The model under review builds one solid part; all positions refer to its coordinate system, in mm. A direction names the side the tool comes from. Give positions to 0.01 mm unless a question says otherwise; leave off trailing zeros. Write each loop counter-clockwise with the first axis right and the second up, starting at its lowest first coordinate (ties: lowest second). Pieces come first, ordered by that corner, then holes.
from build123d import *

# Parameters (mm, degrees)
F0_W        = 70
F0_H        = 40
F0_R        = 2.5
F1_DEPTH    = 5
F2_R        = 10
F3_T1_DEPTH = 65


# Not quite as in the source:
# - a fillet or chamfer that OpenCascade refuses, or shapes differently, is made with other operations: its cross-section is extruded or revolved along the edge and cut away or added


with BuildPart() as f1:
    # F0 (on Top) → F1 (new body)
    with BuildSketch(Plane.XY):
        Rectangle(F0_W, F0_H)
        with Locations((-30, 0)):
            Circle(F0_R, mode=Mode.SUBTRACT)
        with BuildLine():
            ThreePointArc((-25, 12.5), (-24.267766953, 14.267766953), (-22.5, 15))
            Line((-22.5, 15), (-21.7131334842, 15))
            ThreePointArc((-21.7131334842, 15), (-19.9453665312, 14.267766953), (-19.2131334842, 12.5))
            Line((-19.2131334842, 12.5), (-19.2131334842, -12.5))
            ThreePointArc((-19.2131334842, -12.5), (-19.9453665312, -14.267766953), (-21.7131334842, -15))
            Line((-21.7131334842, -15), (-22.5, -15))
            ThreePointArc((-22.5, -15), (-24.267766953, -14.267766953), (-25, -12.5))
            Line((-25, -12.5), (-25, 12.5))
        make_face(mode=Mode.SUBTRACT)
        with BuildLine():
            Line((-14, -12.5), (-14, 12.5))
            ThreePointArc((-14, 12.5), (-13.267766953, 14.267766953), (-11.5, 15))
            Line((-11.5, 15), (-10.7131334842, 15))
            ThreePointArc((-10.7131334842, 15), (-8.9453665312, 14.267766953), (-8.2131334842, 12.5))
            Line((-8.2131334842, 12.5), (-8.2131334842, -12.5))
            ThreePointArc((-8.2131334842, -12.5), (-8.9453665312, -14.267766953), (-10.7131334842, -15))
            Line((-10.7131334842, -15), (-11.5, -15))
            ThreePointArc((-11.5, -15), (-13.267766953, -14.267766953), (-14, -12.5))
        make_face(mode=Mode.SUBTRACT)
        with BuildLine():
            Line((-3, -12.5), (-3, 12.5))
            ThreePointArc((-3, 12.5), (-2.267766953, 14.267766953), (-0.5, 15))
            Line((-0.5, 15), (0.2868665158, 15))
            ThreePointArc((0.2868665158, 15), (2.0546334688, 14.267766953), (2.7868665158, 12.5))
            Line((2.7868665158, 12.5), (2.7868665158, -12.5))
            ThreePointArc((2.7868665158, -12.5), (2.0546334688, -14.267766953), (0.2868665158, -15))
            Line((0.2868665158, -15), (-0.5, -15))
            ThreePointArc((-0.5, -15), (-2.267766953, -14.267766953), (-3, -12.5))
        make_face(mode=Mode.SUBTRACT)
        with BuildLine():
            Line((8, -12.5), (8, 12.5))
            ThreePointArc((8, 12.5), (8.732233047, 14.267766953), (10.5, 15))
            Line((10.5, 15), (11.2868665158, 15))
            ThreePointArc((11.2868665158, 15), (13.0546334688, 14.267766953), (13.7868665158, 12.5))
            Line((13.7868665158, 12.5), (13.7868665158, -12.5))
            ThreePointArc((13.7868665158, -12.5), (13.0546334688, -14.267766953), (11.2868665158, -15))
            Line((11.2868665158, -15), (10.5, -15))
            ThreePointArc((10.5, -15), (8.732233047, -14.267766953), (8, -12.5))
        make_face(mode=Mode.SUBTRACT)
        with BuildLine():
            Line((19, -12.5), (19, 12.5))
            ThreePointArc((19, 12.5), (19.732233047, 14.267766953), (21.5, 15))
            Line((21.5, 15), (22.2868665158, 15))
            ThreePointArc((22.2868665158, 15), (24.0546334688, 14.267766953), (24.7868665158, 12.5))
            Line((24.7868665158, 12.5), (24.7868665158, -12.5))
            ThreePointArc((24.7868665158, -12.5), (24.0546334688, -14.267766953), (22.2868665158, -15))
            Line((22.2868665158, -15), (21.5, -15))
            ThreePointArc((21.5, -15), (19.732233047, -14.267766953), (19, -12.5))
        make_face(mode=Mode.SUBTRACT)
        with Locations((30, 0)):
            Circle(F0_R, mode=Mode.SUBTRACT)
    extrude(amount=F1_DEPTH)

    # F2
    f2_edges = [f1.edges().sort_by_distance(p)[0] for p in [
        (-35, 20, 2.5),
        (-35, -20, 2.5),
        (35, -20, 2.5),
        (35, 20, 2.5),
    ]]
    fillet(f2_edges, radius=F2_R)

    # F3: fillet of radius 3 on 2 edges, made by hand

    # F3_s2 → F3_t1 (cut)
    with BuildSketch(Plane.YZ.offset(-32.5)):
        with BuildLine():
            ThreePointArc((-17, 5), (-19.1213203436, 4.1213203436), (-20, 2))
            Line((-20, 2), (-20, 5))
            Line((-20, 5), (-17, 5))
        make_face()
        with BuildLine():
            ThreePointArc((20, 2), (19.1213203436, 4.1213203436), (17, 5))
            Line((17, 5), (20, 5))
            Line((20, 5), (20, 2))
        make_face()
    extrude(amount=F3_T1_DEPTH, mode=Mode.SUBTRACT)


solid = f1.part
1) Consider section D-D, the plane x = -17. Give the boundary of the cut face in (y, z).
2) Consider section B-B, the plane y = 0. State how many separate pieces and enclosed holes the cut face has, then the cut area to 3 significant figures.
3) Consider section A-A, the plane y = 4.5. Give the boundary of the cut face in (x, z), then the cut area to 3 significant figures.
4) Tool access review of faces 1 (the cylindrical face through (-32.15, 16.99, 2.54)), 2 (the cylindrical face through (-24.248, -14.287, 2.465)): name each direction out of +Z, -Z, +X, -X, +Y, -Y from which nothing blocks a thin tool from reaching the whole face with its end or side.
5) Consider section C-C, the plane x = 20.5. Give the boundary of the cut face in (y, z).
6) To check wall thickness, follow probe 1 along X at (y, z) = (-10, 3.25); probe 2 along X at (y, z) = (-11, 1.95); probe 3 along Y at (x, z) = (11.5, 0.4). State the ranges of each line that lie inside material, in increasing order.
7) Insertion check: pin 1 (0.9 mm diameter, centred on x = 11, z = 3.5, fed in from +Y); pin 2 (6 mm diameter, centred on x = -10.5, y = 13, fed in from -Z). Each pin has a flat end and moves straight along its axis. Give the tip position at first contact, or say it passes through.
Answer block:
1. outline: (-20, 0) - (20, 0) - (20, 2) arc R3 ccw to (17, 5) - (-17, 5) arc R3 ccw to (-20, 2) - close
2. separate pieces: 8
2. enclosed holes: 0
2. area: 155 mm2
3. outline: (-35, 0) - (-25, 0) - (-25, 5) - (-35, 5) - close; (-19.21, 0) - (-14, 0) - (-14, 5) - (-19.21, 5) - close; (-8.21, 0) - (-3, 0) - (-3, 5) - (-8.21, 5) - close; (2.79, 0) - (8, 0) - (8, 5) - (2.79, 5) - close; (13.79, 0) - (19, 0) - (19, 5) - (13.79, 5) - close; (24.79, 0) - (35, 0) - (35, 5) - (24.79, 5) - close
3. area: 205 mm2
4. face 1: +Z, -Z, -X, +Y
4. face 2: +Z, -Z
5. outline: (-20, 0) - (-14.79, 0) - (-14.79, 5) - (-17, 5) arc R3 ccw to (-20, 2) - close; (14.79, 0) - (20, 0) - (20, 2) arc R3 ccw to (17, 5) - (14.79, 5) - close
6. probe 1: x = -35 to -25, -19.21 to -14, -8.21 to -3, 2.79 to 8, 13.79 to 19, 24.79 to 35
6. probe 2: x = -34.95 to -25, -19.21 to -14, -8.21 to -3, 2.79 to 8, 13.79 to 19, 24.79 to 34.95
6. probe 3: y = -20 to -14.99, 14.99 to 20
7. pin 1: stops at y = 19.81
7. pin 2: stops at z = 0
